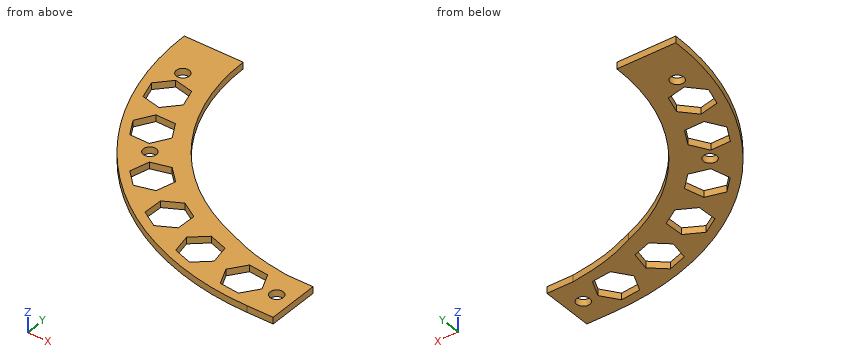
```python
from build123d import *

# Parameters (mm, degrees)
BOSS_EXTRUDE1_DEPTH = 6.35
CUT_EXTRUDE1_REACH  = 8.35
SKETCH3_R           = 6.35
CUT_EXTRUDE2_REACH  = 8.35
SKETCH4_R           = 6.35
BOSS_EXTRUDE2_DEPTH = 6.35
CUT_EXTRUDE4_DEPTH  = 7.3500001


with BuildPart() as part:
    # Sketch1 → Boss-Extrude1 (new body)
    with BuildSketch(Plane.XY):
        with BuildLine():
            Line((0, -203.2), (25.4, -203.2))
            Line((25.4, -203.2), (25.4, -254))
            Line((25.4, -254), (0, -254))
            ThreePointArc((0, -254), (-179.605122421, -179.605122421), (-254, 0))
            Line((-254, 0), (-203.2, 0))
            ThreePointArc((-203.2, 0), (-143.684097937, -143.684097937), (0, -203.2))
        make_face()
    extrude(amount=BOSS_EXTRUDE1_DEPTH)

    # Sketch3 → Cut-Extrude1 (cut, up to next)
    with BuildSketch(Plane.XY.offset(6.35), mode=Mode.PRIVATE) as cut_extrude1_sk1:
        with Locations((-182.568077597, -137.574914293)):
            Circle(SKETCH3_R)
    cut_extrude1_tool1 = extrude(cut_extrude1_sk1.sketch, amount=-CUT_EXTRUDE1_REACH, mode=Mode.PRIVATE) & part.part
    add(cut_extrude1_tool1.solids().sort_by_distance((-182.568078, -137.574914, 6.35))[0], mode=Mode.SUBTRACT)
    # Sketch3 → Cut-Extrude1 (cut, up to next)
    with BuildSketch(Plane.XY.offset(6.35), mode=Mode.PRIVATE) as cut_extrude1_sk2:
        with Locations((-225.127052339, -39.695973415)):
            Circle(SKETCH3_R)
    cut_extrude1_tool2 = extrude(cut_extrude1_sk2.sketch, amount=-CUT_EXTRUDE1_REACH, mode=Mode.PRIVATE) & part.part
    add(cut_extrude1_tool2.solids().sort_by_distance((-225.127052, -39.695973, 6.35))[0], mode=Mode.SUBTRACT)

    # Sketch4 → Cut-Extrude2 (cut, up to next)
    with BuildSketch(Plane.XY.offset(6.35), mode=Mode.PRIVATE) as cut_extrude2_sk1:
        with Locations((9.525, -228.6)):
            Circle(SKETCH4_R)
    cut_extrude2_tool1 = extrude(cut_extrude2_sk1.sketch, amount=-CUT_EXTRUDE2_REACH, mode=Mode.PRIVATE) & part.part
    add(cut_extrude2_tool1.solids().sort_by_distance((9.525, -228.6, 6.35))[0], mode=Mode.SUBTRACT)

    # Sketch5 → Boss-Extrude2 (add)
    with BuildSketch(Plane.XY.offset(6.35)):
        with BuildLine():
            Line((-196.85, 0), (-203.2, 0))
            ThreePointArc((-203.2, 0), (-143.684097937, -143.684097937), (0, -203.2))
            add(Edge.make_bspline(
                [(0, -203.2), (-42.738576364, -198.027670234), (-55.377716847, -189.330212239), (-67.326665214, -184.978492402)],
                knots=[0, 0, 0, 0, 1, 1, 1, 1], degree=3))
            ThreePointArc((-67.326665214, -184.978492402), (-161.250079918, -112.908521496), (-196.85, 0))
        make_face()
    extrude(amount=-BOSS_EXTRUDE2_DEPTH)

    # Sketch8 → Cut-Extrude4 (cut, through all)
    with BuildSketch(Plane.XY.offset(6.35)):
        Polygon((-189.550744798, -129.195114639), (-179.886192663, -112.778692007), (-189.270955635, -96.200733026), (-208.320270741, -96.039196678), (-217.984822875, -112.45561931), (-208.600059904, -129.033578291), align=None)
        Polygon((-212.312705004, -86.857226492), (-199.439243548, -72.815271852), (-205.163202257, -54.645549875), (-223.760622423, -50.51778254), (-236.634083879, -64.559737181), (-230.91012517, -82.729459157), align=None)
        Polygon((-147.628804374, -175.575051243), (-142.755562385, -157.158916673), (-156.267781768, -143.730498026), (-174.65324314, -148.71821395), (-179.526485129, -167.134348521), (-166.014265746, -180.562767167), align=None)
        Polygon((-104.315468483, -204.301604338), (-103.713008923, -185.261133166), (-119.901310879, -175.219152296), (-136.692072394, -184.217642598), (-137.294531954, -203.258113771), (-121.106229998, -213.300094641), align=None)
        Polygon((-55.647161568, -222.540459039), (-59.346411332, -203.853082252), (-77.379779242, -197.713038129), (-91.713897388, -210.260370793), (-88.014647624, -228.94774758), (-69.981279714, -235.087791703), align=None)
        Polygon((-4.122241516, -229.355334852), (-11.933301871, -211.980357553), (-30.886003779, -210.057445601), (-42.027645333, -225.509510947), (-34.216584978, -242.884488246), (-15.26388307, -244.807400198), align=None)
    extrude(amount=-CUT_EXTRUDE4_DEPTH, mode=Mode.SUBTRACT)


solid = part.part
```
Could you check a few things on this model? Use its own coordinates, in mm. Round coordinates to 2 decimals unless told otherwise and drop trailing zeros.
Q1. For P1, Ø16.5, axis at x = 9.525, y = -228.6, coming from the -Z side; P2, Ø7.5, axis at x = -225.13, y = -39.7, coming from the +Z side; P3, Ø1, axis at x = -164.5, z = 3, coming from the +Y side; P4, Ø1.5, axis at x = -77, z = 2.5, coming from the -Y side, each with a flat end and sliding along its axis, tell me the tip position at first contact or that it passes through.
Q2. I want a section at A-A (z = 4). Give the number of separate pieces and of enclosed holes in the cut face, and give its area (3 significant figures).
Q3. Please list where these lines run through material, in increasing order: L1, parallel to Y at x = -229, z = 1.5; L2, parallel to Y at x = -221.5, z = 0.5; L3, parallel to Y at x = 4.5, z = 0.75.
Answer below:
1. P1: stops at z = 0
1. P2: passes through
1. P3: stops at y = -107.35
1. P4: stops at y = -242.28
2. separate pieces: 1
2. enclosed holes: 9
2. area: 15,300 mm2
3. L1: y = -109.89 to -83.15, -56.23 to -44.73, -34.66 to 0
3. L2: y = -124.31 to -84.82, -51.02 to -44.91, -34.48 to 0
3. L3: y = -254 to -232.48, -224.72 to -203.2
